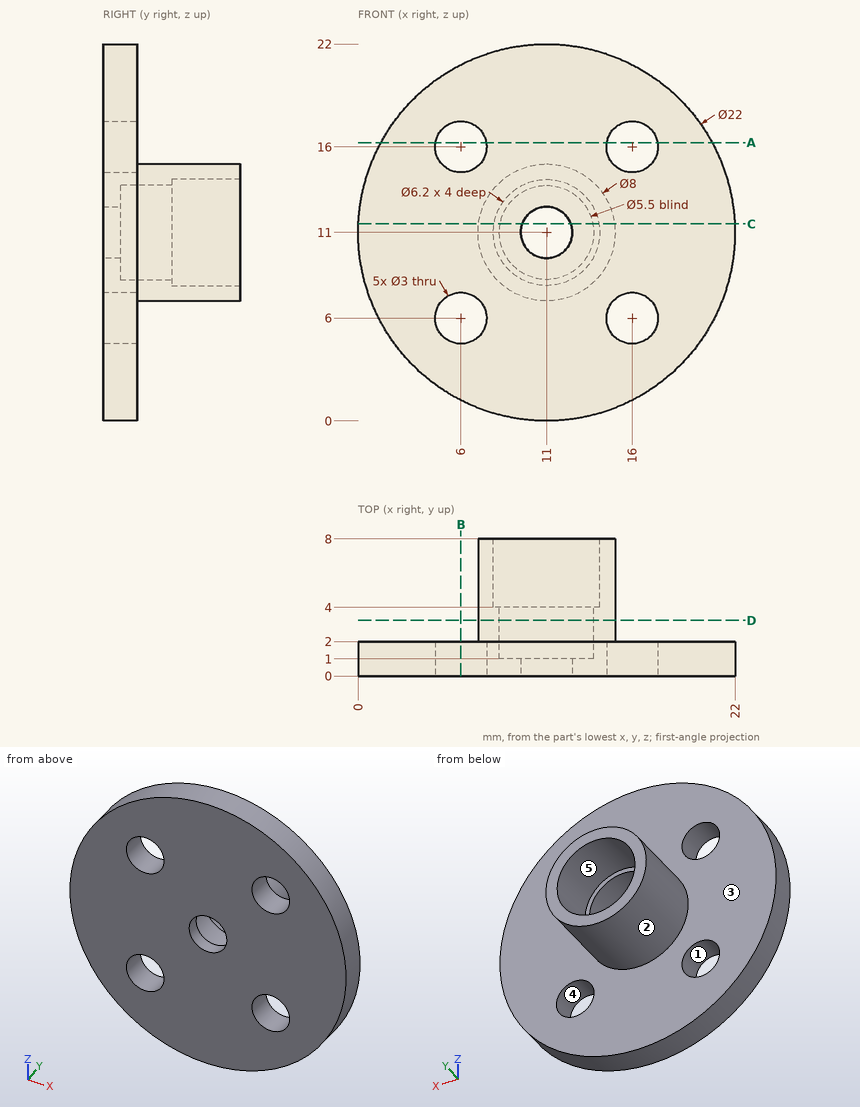
Check sheet for the drawn part. Datum: minimum x, y, z corner. Units: mm. A direction names the side the tool comes from. Give positions to 0.01 mm unless a question says otherwise; leave off trailing zeros. Write each loop counter-clockwise with the first axis right and the second up, starting at its lowest first coordinate (ties: lowest second). Pieces come first, ordered by that corner, then holes. Notation, with made-up numbers: M -29,51 L 17,51 A20 cw 17,87 Z; hole C 31,-16.5 d7. An arc over 180 degrees is marked long. One line per question, with ' | ' between items.
1) Section check A-A on z = 16.25. Enter the section's corners in (x, y), plus the area to 3 significant figures.
Result:
outline: M 1.33,0 L 4.52,0 L 4.52,2 L 1.33,2 Z; M 7.48,0 L 14.52,0 L 14.52,2 L 7.48,2 Z; M 17.48,0 L 20.67,0 L 20.67,2 L 17.48,2 Z | area: 26.8 mm2
2) Set-up check for the marked faces 4 and 5: record each of +Z, -Z, +X, -X, +Y, -Y from which the full face is reachable in a straight line by a thin tool's end or side.
Result:
face 4: +Y, -Y | face 5: +Y
3) Section check C-C on z = 11.5. Enter the section's corners in (x, y), plus the area to 3 significant figures.
Result:
outline: M 0.01,0 L 9.59,0 L 9.59,1 L 8.3,1 L 8.3,4 L 7.94,4 L 7.94,8 L 7.03,8 L 7.03,2 L 0.01,2 Z; M 12.41,0 L 21.99,0 L 21.99,2 L 14.97,2 L 14.97,8 L 14.06,8 L 14.06,4 L 13.7,4 L 13.7,1 L 12.41,1 Z | area: 48.0 mm2
4) Thickness scan on line 1 along X through (y, z) = (0.6, 11); line 2 along X through (y, z) = (0.5, 16); line 3 along Y through (x, z) = (10.25, 4.25). Record the ranges inside material, lowest first. Write a range as [from, to].
Result:
line 1: x = [0, 9.5], [12.5, 22] | line 2: x = [1.2, 4.5], [7.5, 14.5], [17.5, 20.8] | line 3: y = [0, 2]
5) Section check D-D on y = 3.25. Enter the section's corners in (x, z).
Result:
outline: C 11,11 d8; hole C 11,11 d5.5
6) Mould release check, pull along Z, two halves, no side actions. Record for the marked faces 1, 2 and 3: released by +Z, released by -Z, zero draft, split by the parting line, or undercut.
Result:
face 1: undercut | face 2: split by the parting line | face 3: zero draft
7) Section check B-B on x = 6. Enter the section's corners in (y, z).
Result:
outline: M 0,1.2 L 2,1.2 L 2,4.5 L 0,4.5 Z; M 0,7.5 L 2,7.5 L 2,14.5 L 0,14.5 Z; M 0,17.5 L 2,17.5 L 2,20.8 L 0,20.8 Z
8) Gauge pin test, flat ends, axial feed: pin 1 Ø3 at (x, z) = (10, 11) entering from +Y; pin 2 Ø2.5 at (x, z) = (6, 16) entering from -Y; pin 3 Ø1.5 at (x, y) = (19, 2) entering from -Z; pin 4 Ø3.5 at (x, z) = (16, 6) entering from +Y. Record the tip position at first contact, or that the pin passes through.
Result:
pin 1: stops at y = 1 | pin 2: passes through | pin 3: stops at z = 2.73 | pin 4: stops at y = 2
